```python
from build123d import *

# Parameters (mm, degrees)
BOSS_EXTRU_1_DEPTH      = 6.35
ESQUISSE2_W             = 401.8
ESQUISSE2_H             = 6.35
ENL_V_MAT_EXTRU_1_DEPTH = 643.307344657
D_GAGEMENT_1_41_D       = 7.14248
ESQUISSE5_W             = 401.8
ESQUISSE5_H             = 1.35
BOSS_EXTRU_2_DEPTH      = 6.35


with BuildPart() as part:
    # Esquisse1 → Boss.-Extru.1 (new body)
    with BuildSketch(Plane.XY):
        Polygon((-615.95, 52.7), (-615.95, -52.7), (-553.8, -52.7), (-553.8, -113.5), (-493, -113.5), (-493, -174.3), (-91.2, -174.3), (-91.2, -113.5), (-30.4, -113.5), (-30.4, -52.7), (0, -52.7), (0, 52.7), (-30.4, 52.7), (-30.4, 113.5), (-91.2, 113.5), (-91.2, 182), (-493, 182), (-493, 113.5), (-553.8, 113.5), (-553.8, 52.7), align=None)
    extrude(amount=BOSS_EXTRU_1_DEPTH)

    # Esquisse2 → Enlèv. mat.-Extru.1 (cut, through all)
    with BuildSketch(Plane.XY.offset(6.35)):
        with Locations((-292.1, 178.825)):
            Rectangle(ESQUISSE2_W, ESQUISSE2_H)
    extrude(amount=-ENL_V_MAT_EXTRU_1_DEPTH, mode=Mode.SUBTRACT)

    # Dégagement 1/41 (through all)
    with Locations(Plane(origin=(0, 0, 0), x_dir=(-1, 0, 0), z_dir=(0, 0, -1))):
        with Locations((45.6, 98.3), (45.6, -98.3), (538.6, -98.3), (538.6, 98.3)):
            Hole(D_GAGEMENT_1_41_D / 2)

    # Esquisse5 → Boss.-Extru.2 (add, through all)
    with BuildSketch(Plane.XY.offset(6.35)):
        with Locations((-292.1, -174.975)):
            Rectangle(ESQUISSE5_W, ESQUISSE5_H)
    extrude(amount=-BOSS_EXTRU_2_DEPTH)


with BuildPart() as body_2:
    # Symétrie1: mirrored copy
    add(part.part.mirror(Plane(origin=(0, -52.7, 6.35), x_dir=(0, 0, 1), z_dir=(-1, 0, 0))))


solid = body_2.part
```
Part model, mm, in its own coordinate system. Round coordinates to 2 decimals unless told otherwise and drop trailing zeros. Loops run counter-clockwise (first coordinate to the right, second up) from the corner with the lowest first, then second, coordinate; pieces in that order, holes last. Notation, with made-up numbers: (77.25, 39.5) -> (131.25, 39.5) arc R25 cw to (131.25, 61.5) -> close; hole circle Ø5 at (-30.75, 34). An arc over 180 degrees is marked (long way). Use one line per item in the form item = value. Start each with the question number.
Item 1: Band-saw the part on B-B (y = -138). List the corners of the cut face in (x, z).
Item 2: Band-saw the part on A-A (z = 5.25). List the corners of the cut face in (x, y).
Item 3: Drill centre lines: line 1 along Y through (x, z) = (538.6, 4.5); line 2 along Y through (x, z) = (575, 1.5); line 3 along X through (y, z) = (122, 1.5). Where is each one in solid material? Low to high.
Item 4: Band-saw the part on C-C (y = 89). List the corners of the cut face in (x, z), plus the area to 3 significant figures.
Item 5: Drop flat-ended pins along their axis: pin 1 Ø8 at (x, y) = (478, -15) entering from -Z; pin 2 Ø3 at (y, z) = (-132, 3) entering from -X; pin 3 Ø1.9 at (x, z) = (57.5, 1.5) entering from -Y; pin 4 Ø3 at (y, z) = (75, 3) entering from -X. Give the stop position or say it passes through.
Data:
q1.outline = (91.2, 0) -> (493, 0) -> (493, 6.35) -> (91.2, 6.35) -> close
q2.outline = (0, -52.7) -> (30.4, -52.7) -> (30.4, -113.5) -> (91.2, -113.5) -> (91.2, -175.65) -> (493, -175.65) -> (493, -113.5) -> (553.8, -113.5) -> (553.8, -52.7) -> (615.95, -52.7) -> (615.95, 52.7) -> (553.8, 52.7) -> (553.8, 113.5) -> (493, 113.5) -> (493, 175.65) -> (91.2, 175.65) -> (91.2, 113.5) -> (30.4, 113.5) -> (30.4, 52.7) -> (0, 52.7) -> close; hole circle Ø7.14 at (45.6, -98.3); hole circle Ø7.14 at (45.6, 98.3); hole circle Ø7.14 at (538.6, -98.3); hole circle Ø7.14 at (538.6, 98.3)
q3.line_1 = -113.5 to -101.87, -94.73 to 94.73, 101.87 to 113.5
q3.line_2 = -52.7 to 52.7
q3.line_3 = 91.2 to 493
q4.outline = (30.4, 0) -> (553.8, 0) -> (553.8, 6.35) -> (30.4, 6.35) -> close
q4.area = 3,320 mm^2
q5.pin_1 = 0
q5.pin_2 = 91.2
q5.pin_3 = -113.5
q5.pin_4 = 30.4
